```python
from build123d import *

# Parameters (mm, degrees)
F0_W      = 96
F0_H      = 36
F1_DEPTH  = 12
F2_R      = 3.6
F3_DEPTH  = 12.001
F5_DEPTH  = 12.001
F8_DEPTH  = 10
F9_R      = 6
F10_DEPTH = 10.001


with BuildPart() as f1:
    # F0 (on Top) → F1 (new body)
    with BuildSketch(Plane.XY):
        with Locations((-48, 18)):
            Rectangle(F0_W, F0_H)
    extrude(amount=F1_DEPTH)

    # F2 (on face) → F3 (cut, through all)
    with BuildSketch(Plane.XY.offset(12)):
        with Locations((-12, 12)):
            Circle(F2_R)
        with Locations((-84, 12)):
            Circle(F2_R)
    extrude(amount=-F3_DEPTH, mode=Mode.SUBTRACT)

    # F4 (on face) → F5 (cut, through all)
    with BuildSketch(Plane.XY.offset(12)):
        with BuildLine():
            Line((-41.0088156365, -1.4656213384), (-41.0088156365, 14.6488003482))
            ThreePointArc((-41.0088156365, 14.6488003482), (-47.8732599834, 21.9988525465), (-54.9993160638, 14.9021499143))
            Line((-54.9993160638, 14.9021499143), (-54.9993160638, -1.4656213384))
            Line((-54.9993160638, -1.4656213384), (-41.0088156365, -1.4656213384))
        make_face()
    extrude(amount=-F5_DEPTH, mode=Mode.SUBTRACT)

    # F7 (on offset) → F8 (join)
    with BuildSketch(Plane(origin=(0, 36, 0), x_dir=(-1, 0, 0), z_dir=(0, 1, 0))):
        with BuildLine():
            Line((35.7998133379, 40.8387265113), (0, 11.9867287576))
            Line((0, 11.9867287576), (96, 11.9867287576))
            Line((96, 11.9867287576), (60.2001866621, 40.8387265113))
            ThreePointArc((60.2001866621, 40.8387265113), (48, 46), (35.7998133379, 40.8387265113))
        make_face()
    extrude(amount=-F8_DEPTH)

    # F9 (on face) → F10 (cut, through all)
    with BuildSketch(Plane.XZ.offset(-26)):
        with Locations((-48, 27)):
            Circle(F9_R)
    extrude(amount=-F10_DEPTH, mode=Mode.SUBTRACT)


solid = f1.part
```
Check sheet for the modelled part. Datum: model origin and axes. Units: mm. A direction names the side the tool comes from. Coordinates: 2 decimals unless noted, no trailing zeros. Order: outer loops, then holes, each group sorted by start corner. A loop starts at its lowest first (then second) coordinate and runs counter-clockwise, first axis right, second up. Notation, with made-up numbers: (-15.5, -28.5) -> (15.5, -28.5) arc R18 cw to (15.5, 3.5) -> close; hole circle Ø4 at (-1.75, 83). An arc over 180 degrees is marked (long way). Write each question's results on one line, items separated by ' | '. Start each with the question number.
1) Section check A-A (x = -48). Enter the section's corners in (y, z).
2) Material ranges on line 1 along Y through (x, z) = (-84, 3); line 2 along Z through (x, y) = (-48, 29); line 3 along X through (y, z) = (11, 3.5), recorded low to high.
3) Section check D-D (y = 5). Enter the section's corners in (x, z).
4) Section check C-C (z = 9). Enter the section's corners in (x, y).
5) Section check B-B (y = 12). Enter the section's corners in (x, z), and give its area (3 significant figures).
6) Draft check along Y on faces 4 (the face through (-41.009, 7, 6)), 5 (the face through (-82.339, 8.806, 6.084)), 6 (the face through (-47, 26, 18)). Enter one of: pulls with the +Y half, pulls with the -Y half, needs draft (parallel to the pull), parting line crosses it, or undercut.
7) Depth check by flat-ended pin: pin 1 (6 mm diameter, centred on x = -86.5, y = 16.5, fed in from +Z); pin 2 (10 mm diameter, centred on x = -73.5, z = 34.5, fed in from -Y). Enter the tip coordinate at first touch or a pass-through.
8) Set-up check for faces 1 (the face through (-48.7, 22.3, 12)), 2 (the face through (0, 18, 6)), 3 (the face through (-54.999, 8, 6)): record each of +Z, -Z, +X, -X, +Y, -Y from which the full face is reachable in a straight line by a thin tool's end or side.
Checked values:
1) outline: (22, 0) -> (36, 0) -> (36, 21) -> (26, 21) -> (26, 12) -> (22, 12) -> close; (26, 33) -> (36, 33) -> (36, 46) -> (26, 46) -> close
2) line 1: 0 to 8.4, 15.6 to 36 | line 2: 0 to 21, 33 to 46 | line 3: -96 to -87.46, -80.54 to -55, -41.01 to -15.46, -8.54 to 0
3) outline: (-96, 0) -> (-55, 0) -> (-55, 12) -> (-96, 12) -> close; (-41.01, 0) -> (0, 0) -> (0, 12) -> (-41.01, 12) -> close
4) outline: (-96, 0) -> (-55, 0) -> (-55, 14.9) arc R7 cw (long way) to (-41.01, 14.65) -> (-41.01, 0) -> (0, 0) -> (0, 36) -> (-96, 36) -> close; hole circle Ø7.2 at (-84, 12); hole circle Ø7.2 at (-12, 12)
5) outline: (-96, 0) -> (-87.6, 0) -> (-87.6, 12) -> (-96, 12) -> close; (-80.4, 0) -> (-55, 0) -> (-55, 12) -> (-80.4, 12) -> close; (-41.01, 0) -> (-15.6, 0) -> (-15.6, 12) -> (-41.01, 12) -> close; (-8.4, 0) -> (0, 0) -> (0, 12) -> (-8.4, 12) -> close | area: 811 mm²
6) face 4: needs draft | face 5: undercut | face 6: pulls with the -Y half
7) pin 1: z = 12 | pin 2: y = 26
8) face 1: +Z, +X, -X, -Y | face 2: +Z, -Z, +X, +Y, -Y | face 3: +Z, -Z, -Y
